Read the model definition and answer for the solid it produces. Units are mm, in the model's axes. A direction names the side the tool comes from. Round coordinates to 2 decimals unless told otherwise and drop trailing zeros. Loops run counter-clockwise (first coordinate to the right, second up) from the corner with the lowest first, then second, coordinate; pieces in that order, holes last. Notation, with made-up numbers: M -23.75,48 L -15.75,48 A19 ccw -15.75,75 Z; hole C -31.75,89.25 d9. An arc over 180 degrees is marked long. Answer as CSV lines item,"result".
Autodesk Inventor part; units mm, degrees
ref_plane "YZ Plane" through (0, 0, 0) normal (1, 0, 0) x (0, 1, 0)
ref_plane "XZ Plane" through (0, 0, 0) normal (0, 1, 0) x (-1, 0, 0)
ref_plane "XY Plane" through (0, 0, 0) normal (0, 0, 1) x (1, 0, 0)
sketch "Sketch1" plane through (0, 0, 0) normal (0, 0, 1) x (1, 0, 0)
  circle A0 centre (0, 13.5) radius 2
  circle A1 centre (-100, 13.5) radius 2
  line L0 (-100, 13.5) -> (-105, 13.5) construction
  line L1 (-100, 13.5) -> (-95, 13.5) construction
  line L2 (-105, 13.5) -> (-105, 8.5) construction
  line L3 (-105, 8.5) -> (-95, 8.5)
  line L4 (-95, 8.5) -> (-95, 18.5)
  line L5 (-95, 18.5) -> (-105, 18.5)
  line L6 (-105, 18.5) -> (-105, 8.5)
  line L7 (-5, 8.5) -> (5, 8.5)
  line L8 (5, 8.5) -> (5, 18.5)
  line L9 (5, 18.5) -> (-5, 18.5)
  line L10 (-5, 18.5) -> (-5, 8.5)
  line L11 (-5, 8.5) -> (5, 18.5) construction
  line L12 (5, 8.5) -> (-5, 18.5) construction
  point P0 (0, 0)
  dimension "d0" = 5
  dimension "d1" = 180
  dimension "d2" = 5
  dimension "d3" = 90
  dimension "d4" = 10
  dimension "d5" = 10
  dimension "d6" = 10
  dimension "d7" = 10
extrude "Extrusion1" add sketch "Sketch1" along normal blind 10
sketch "Sketch2" plane through (0, 0, 10) normal (0, 0, 1) x (1, 0, 0)
  circle A0 centre (-100, 13.5) radius 2
  line L0 (-105, 8.5) -> (-95, 8.5)
  line L1 (-95, 8.5) -> (-95, 18.5)
  line L2 (-95, 18.5) -> (-105, 18.5) construction
  line L3 (-105, 18.5) -> (-105, 8.5)
  line L4 (-92.5, 21) -> (-107.5, 21) construction
  line L5 (-107.5, 21) -> (-107.5, 6) construction
  line L6 (-107.5, 6) -> (-92.5, 6) construction
  line L7 (-92.5, 6) -> (-92.5, 21) construction
  circle A1 centre (-100, 13.5) radius 2 construction
  line L8 (-92.5, 21) -> (-107.5, 6) construction
  line L9 (-107.5, 21) -> (-92.5, 6) construction
  line L10 (-107.5, 6) -> (7.5, 6)
  line L11 (7.5, 6) -> (7.5, 71)
  line L12 (7.5, 71) -> (-107.5, 71)
  line L13 (-107.5, 71) -> (-107.5, 6)
  circle A2 centre (0, 13.5) radius 2
  point P0 (0, 0)
  dimension "d10" = 15
  dimension "d11" = 15
  dimension "d12" = 115
  dimension "d13" = 65
extrude "Extrusion2" add sketch "Sketch2" along normal blind 10
sketch "Sketch3" plane through (0, 0, 20) normal (0, 0, 1) x (1, 0, 0)
  circle A0 centre (-100, 13.5) radius 2 construction
  circle A1 centre (0, 13.5) radius 2 construction
  line L0 (-103.6, 17.1) -> (-96.4, 17.1)
  line L1 (-96.4, 17.1) -> (-96.4, 9.9)
  line L2 (-96.4, 9.9) -> (-103.6, 9.9)
  line L3 (-103.6, 9.9) -> (-103.6, 17.1)
  line L4 (-103.6, 17.1) -> (-96.4, 9.9) construction
  line L5 (-96.4, 17.1) -> (-103.6, 9.9) construction
  line L6 (-3.6, 17.1) -> (3.6, 17.1)
  line L7 (3.6, 17.1) -> (3.6, 9.9)
  line L8 (3.6, 9.9) -> (-3.6, 9.9)
  line L9 (-3.6, 9.9) -> (-3.6, 17.1)
  line L10 (-3.6, 17.1) -> (3.6, 9.9) construction
  line L11 (3.6, 17.1) -> (-3.6, 9.9) construction
  point P0 (0, 0)
  dimension "d16" = 7.2
  dimension "d17" = 7.2
  dimension "d18" = 7.2
  dimension "d19" = 7.2
extrude "Extrusion3" cut sketch "Sketch3" against normal blind 2.5
sketch "Sketch4" plane through (0, 0, 10) normal (0, 0, -1) x (-1, 0, 0)
  line L0 (-7.5, 6) -> (-7.5, 71) construction
  line L1 (-7.5, 71) -> (20, 71) construction
  line L2 (-7.5, 71) -> (107.5, 71) construction
  line L3 (20, 71) -> (23, 71) construction
  line L4 (23, 71) -> (23, 68) construction
  line L5 (23, 68) -> (20, 68) construction
  line L6 (20, 68) -> (20, 71) construction
  line L7 (23, 68) -> (77, 68) construction
  line L8 (77, 68) -> (77, 14) construction
  line L9 (23, 68) -> (23, 41) construction
  line L10 (23, 68) -> (50, 68) construction
  circle A0 centre (77, 68) radius 1.5
  circle A1 centre (77, 14) radius 1.5
  circle A2 centre (23, 68) radius 1.5
  circle A3 centre (23, 41) radius 1.5
  point P0 (0, 0)
  dimension "d22" = 27.5
  dimension "d23" = 3
  dimension "d24" = 3
  dimension "d25" = 54
  dimension "d26" = 54
  dimension "d27" = 90
  dimension "d28" = 27
  dimension "d29" = 90
  dimension "d30" = 3
  dimension "d31" = 3
  dimension "d32" = 3
  dimension "d33" = 3
extrude "Extrusion4" cut sketch "Sketch4" against normal up to surface (10 mm away)
properties part number "base_plate"
1) Find section D-D, the plane x = -48. Give the vertices of the cut face in (y, z).
Evaluation:
outline,"M 6,10 L 71,10 L 71,20 L 6,20 Z"
2) Each of these flat-tipped pins is pushed along its axis until it touches: P1, Ø3, axis at y = 14.5, z = 6.5, coming from the +X side; P2, Ø5, axis at y = 14, z = 5, coming from the -X side; P3, Ø8, axis at x = -99, y = 13.5, coming from the +Z side; P4, Ø1, axis at x = -15.5, y = 19, coming from the -Z side. Where does it stop, or does it pass through?
Evaluation:
P1,"stops at x = 5"
P2,"stops at x = -105"
P3,"stops at z = 20"
P4,"stops at z = 10"
3) Find section B-B, the plane x = 0. Give the vertices of the cut face in (y, z), then the cut area to 3 significant figures.
Evaluation:
outline,"M 6,10 L 8.5,10 L 8.5,0 L 11.5,0 L 11.5,17.5 L 9.9,17.5 L 9.9,20 L 6,20 Z; M 15.5,0 L 18.5,0 L 18.5,10 L 71,10 L 71,20 L 17.1,20 L 17.1,17.5 L 15.5,17.5 Z"
area,"662 mm^2"
4) Find section A-A, the plane z = 6.5. Give the vertices of the cut face in (x, y), then the cut area to 3 significant figures.
Evaluation:
outline,"M -105,8.5 L -95,8.5 L -95,18.5 L -105,18.5 Z; M -5,8.5 L 5,8.5 L 5,18.5 L -5,18.5 Z; hole C -100,13.5 d4; hole C 0,13.5 d4"
area,"175 mm^2"
5) Find section C-C, the plane x = -77. Give the vertices of the cut face in (y, z), then the cut area to 3 significant figures.
Evaluation:
outline,"M 6,10 L 12.5,10 L 12.5,20 L 6,20 Z; M 15.5,10 L 66.5,10 L 66.5,20 L 15.5,20 Z; M 69.5,10 L 71,10 L 71,20 L 69.5,20 Z"
area,"590 mm^2"
6) A tool of negligible diameter and unlimited length cuts with its end or side. For faces 4 (the flat face through (0, 18.5, 5)), 5 (the flat face through (-100, 9.9, 19)), 6 (the flat face through (-5, 14, 5)), 7 (the flat face through (-100, 8.5, 5)), from which of +Z, -Z, +X, -X, +Y, -Y can it reach the whole face along a straight path? Write none if from no direction.
Evaluation:
face 4,"-Z, +X, -X, +Y"
face 5,"+Z"
face 6,"-Z, +Y, -Y"
face 7,"-Z, +X, -X, -Y"
7) Determine the mould class of faces 1 (the flat face through (-107.5, 39, 15)), 2 (the cylindrical face through (-22.675, 39.536, 14.93)), 3 (the flat face through (-100, 18.5, 5)) for opening direction X: released by +X, released by -X, zero draft, split by the parting line, or undercut.
Evaluation:
face 1,"released by -X"
face 2,"undercut"
face 3,"zero draft"
8) Straight lines are drawn through the part: line 1 (X direction, y = 68, z = 16.25); line 2 (Y direction, x = -23, z = 17.75); line 3 (Y direction, x = 0, z = 8). For each, find the intervals that lie inside material, in ascending order.
Evaluation:
line 1,"x = -107.5 to -78.5, -75.5 to -24.5, -21.5 to 7.5"
line 2,"y = 6 to 39.5, 42.5 to 66.5, 69.5 to 71"
line 3,"y = 8.5 to 11.5, 15.5 to 18.5"
